Autodesk Inventor part; units mm, degrees
ref_plane "YZ Plane" through (0, 0, 0) normal (1, 0, 0) x (0, 1, 0)
ref_plane "XZ Plane" through (0, 0, 0) normal (0, 1, 0) x (-1, 0, 0)
ref_plane "XY Plane" through (0, 0, 0) normal (0, 0, 1) x (1, 0, 0)
sketch "Sketch1" plane through (0, 0, 0) normal (0, 0, 1) x (1, 0, 0)
  circle A0 centre (0, 0) radius 3.175
  dimension "d0" = 6.35
extrude "Extrusion1" add sketch "Sketch1" along normal blind 88.9
sketch "Sketch2" plane through (0, 0, 88.9) normal (0, 0, 1) x (1, 0, 0)
  circle A0 centre (0, 0) radius 3.175
  arc A1 (2.7496, 1.5875) -> (-2.7496, 1.5875) centre (0, 0) ccw
  arc A2 (-2.7496, -1.5875) -> (2.7496, -1.5875) centre (0, 0) ccw
  line L0 (2.7496, 1.5875) -> (2.7496, -1.5875)
  line L1 (-2.7496, 1.5875) -> (-2.7496, -1.5875)
  line L2 (0, 3.175) -> (0, -3.175) construction
  dimension "d3" = 3.175
extrude "Extrusion2" add sketch "Sketch2" along normal blind 5.08 contours L0 A0 L1
sketch "Sketch3" plane through (0, 0, 93.98) normal (0, 0, 1) x (1, 0, 0)
  line L0 (-6.35, -6.35) -> (6.35, -6.35)
  line L1 (6.35, -6.35) -> (6.35, 6.35)
  line L2 (6.35, 6.35) -> (-6.35, 6.35)
  line L3 (-6.35, 6.35) -> (-6.35, -6.35)
  line L4 (-6.35, -6.35) -> (6.35, 6.35) construction
  line L5 (6.35, -6.35) -> (-6.35, 6.35) construction
  point P0 (0, 0)
  dimension "d6" = 12.7
extrude "Extrusion3" add sketch "Sketch3" along normal blind 11.176
sketch "Sketch4" plane through (0, 0, 105.156) normal (0, 0, 1) x (1, 0, 0)
  line L0 (6.35, 6.35) -> (-6.35, 6.35)
  line L1 (-6.35, -6.35) -> (6.35, -6.35)
  line L2 (6.35, 6.35) -> (3.175, 6.35)
  line L3 (3.175, 6.35) -> (3.175, -6.35)
  line L4 (3.175, -6.35) -> (6.35, -6.35)
  line L5 (6.35, -6.35) -> (6.35, 6.35)
  line L6 (-6.35, 6.35) -> (-3.175, 6.35)
  line L7 (-3.175, 6.35) -> (-3.175, -6.35)
  line L8 (-3.175, -6.35) -> (-6.35, -6.35)
  line L9 (-6.35, -6.35) -> (-6.35, 6.35)
  line L10 (3.175, 0) -> (-3.175, 0) construction
  point P0 (0, 0)
  point P1 (0, 0)
  dimension "d9" = 6.35
extrude "Extrusion4" add sketch "Sketch4" along normal blind 19.05 contours L5 L1 L3 L0 | L7 L1 L9 L0
sketch "Sketch5" plane through (6.35, -6.35, 93.98) normal (1, 0, 0) x (0, 0, -1)
  line L0 (-30.226, 12.7) -> (-30.226, 0) construction
  line L1 (-30.226, 6.35) -> (-23.876, 6.35) construction
  circle A0 centre (-23.876, 6.35) radius 3.175
  point P0 (93.98, 6.35)
  dimension "d12" = 6.35
  dimension "d13" = 6.35
extrude "Extrusion5" cut sketch "Sketch5" against normal through all
fillet "Fillet1" radius 1.5875 8 edges at (4.7625, 6.35, 124.206) (4.7625, -6.35, 124.206) (-4.7625, -6.35, 124.206) (-4.7625, 6.35, 124.206) (6.35, 0, 93.98) (0, 6.35, 93.98) (-6.35, 0, 93.98) (0, -6.35, 93.98)
properties part number "cylinder piston"
The model under review builds one solid part; all positions refer to its coordinate system, in mm. A direction names the side the tool comes from. Give positions to 0.01 mm unless a question says otherwise; leave off trailing zeros. Order: outer loops, then holes, each group sorted by start corner. A loop starts at its lowest first (then second) coordinate and runs counter-clockwise, first axis right, second up. Notation, with made-up numbers: (-21.5, 21.5) - (4.5, 21.5) arc R11 cw to (4.5, 27.5) - close; hole circle Ø7 at (41.25, 22.25). An arc over 180 degrees is marked (long way). Use CSV: the item, a comma, the result in double quotes. Start each with the question number.
Q1. We need section A-A, the plane y = 0. State how many separate pieces and enclosed holes the cut face has, and give its area (3 significant figures).
Q2. We need section C-C, the plane z = 27. Write out the cut boundary in (x, y) (3 decimals), and give its area (3 significant figures).
Q3. The part is to be moulded in two halves that separate along Z. For faces 4 (the flat face through (-3.175, 0.1, 114.5)), 5 (the flat face through (0, 0, 105.156)), 6 (the cylindrical face through (4.785, 0.14, 121.028)), say which applies: +Z half, -Z half, draft (parallel to the pull), parting line (faces both ways), or undercut.
Q4. Clearance check with flat-ended pins moving along their axes: pin 1 Ø2.5 at (y, z) = (1, 91.5) entering from +X; pin 2 Ø7.5 at (x, y) = (-1, 1.5) entering from -Z; pin 3 Ø1.9 at (x, y) = (1, 0.5) entering from +Z; pin 4 Ø1.6 at (y, z) = (0, 91.5) entering from -X. State where each tip first meets the part, or that it passes through.
Q5. To check wall thickness, follow line 1 along Z through (x, y) = (-1.75, -3); line 2 along Z through (x, y) = (5.75, -0.5); line 3 along X through (y, z) = (0, 77) (3 decimals). State the ranges of each line that lie inside material, in increasing order. Write a range as [from, to].
Q6. Tool access review of faces 1 (the flat face through (2.75, 0, 91)), 2 (the cylindrical face through (-0.69, 3.1, 46.33)), 3 (the flat face through (3.175, 0.1, 114.5)): name each direction out of +Z, -Z, +X, -X, +Y, -Y from which nothing blocks a thin tool from reaching the whole face with its end or side.
Outcome:
1,separate pieces,"3"
1,enclosed holes,"0"
1,area,"814 mm^2"
2,outline,"circle Ø6.35 at (0, 0)"
2,area,"31.7 mm^2"
3,face 4,"draft"
3,face 5,"+Z half"
3,face 6,"undercut"
4,pin 1,"stops at x = 2.75"
4,pin 2,"stops at z = 0"
4,pin 3,"stops at z = 105.16"
4,pin 4,"stops at x = -2.75"
5,line 1,"z = [93.98, 105.16]"
5,line 2,"z = [94.32, 114.72], [120.99, 124.21]"
5,line 3,"x = [-3.175, 3.175]"
6,face 1,"+X, +Y, -Y"
6,face 2,"-Z"
6,face 3,"+Z, +Y, -Y"
